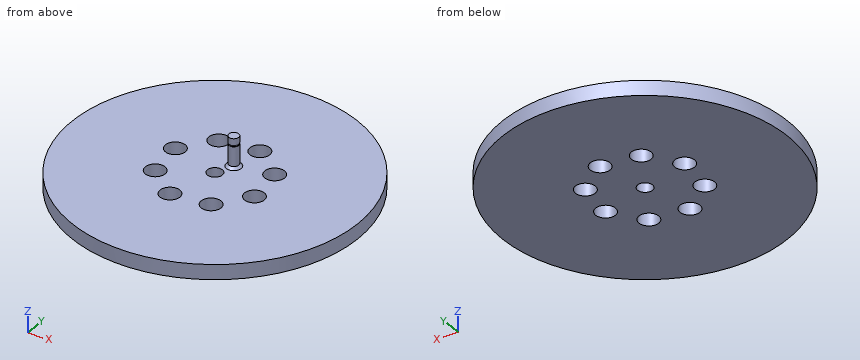
from build123d import *

# Parameters (mm, degrees)
SKETCH_1_R          = 57.5
SKETCH_1_R_2        = 3
EXTRUDE_1_DEPTH     = 6
SKETCH_3_R          = 4
CUT_EXTRUDE_2_DEPTH = 82.538334543
SKETCH_4_R          = 2
EXTRUDE_2_DEPTH     = 12
CUT_EXTRUDE_START   = -3.2
SKETCH_6_R          = 2
SKETCH_6_R_2        = 1.9
CUT_EXTRUDE_3_DEPTH = 0.5
CHAMFER_1_SIZE      = 1


with BuildPart() as part:
    # 草图1 → 凸台-拉伸1 (new body)
    with BuildSketch(Plane.XY):
        Circle(SKETCH_1_R)
        Circle(SKETCH_1_R_2, mode=Mode.SUBTRACT)
    extrude(amount=EXTRUDE_1_DEPTH)

    # 草图3 → 切除-拉伸2 (cut, through all)
    with BuildSketch(Plane(origin=(0, 0, 0), x_dir=(-1, 0, 0), z_dir=(0, 0, -1))):
        with Locations((-5.091227954, 19.341132281)):
            Circle(SKETCH_3_R)
        with Locations((10.076203981, 17.276287603)):
            Circle(SKETCH_3_R)
        with Locations((19.341132281, 5.091227954)):
            Circle(SKETCH_3_R)
        with Locations((17.276287603, -10.076203981)):
            Circle(SKETCH_3_R)
        with Locations((5.091227954, -19.341132281)):
            Circle(SKETCH_3_R)
        with Locations((-10.076203981, -17.276287603)):
            Circle(SKETCH_3_R)
        with Locations((-19.341132281, -5.091227954)):
            Circle(SKETCH_3_R)
        with Locations((-17.276287603, 10.076203981)):
            Circle(SKETCH_3_R)
    extrude(amount=-CUT_EXTRUDE_2_DEPTH, mode=Mode.SUBTRACT)

    # 草图4 → 凸台-拉伸2 (add)
    with BuildSketch(Plane.XY.offset(6)):
        with Locations((2.976659474, 6.884003078)):
            Circle(SKETCH_4_R)
    extrude(amount=EXTRUDE_2_DEPTH)

    # 草图6 → 切除-拉伸3 (cut)
    with BuildSketch(Plane.XY.offset(18).offset(CUT_EXTRUDE_START)):
        with Locations((2.976659474, 6.884003078)):
            Circle(SKETCH_6_R)
        with Locations((2.976659474, 6.884003078)):
            Circle(SKETCH_6_R_2, mode=Mode.SUBTRACT)
    extrude(amount=CUT_EXTRUDE_3_DEPTH, mode=Mode.SUBTRACT)

    # 倒角1
    chamfer_1_edges = [part.edges().sort_by_distance(p)[0] for p in [
        (0.976659474, 6.884003078, 6),
    ]]
    chamfer(chamfer_1_edges, length=CHAMFER_1_SIZE)


solid = part.part
Design review of the part built by this model. Coordinates are the model's own, in mm. Coordinates: 2 decimals unless noted, no trailing zeros. Order: outer loops, then holes, each group sorted by start corner. A loop starts at its lowest first (then second) coordinate and runs counter-clockwise, first axis right, second up. Notation, with made-up numbers: M 62,-11.5 L 95,-11.5 A30 cw 95,22.5 Z; hole C 29,35 d9. An arc over 180 degrees is marked long. Use a Markdown table: item, result.
(1) Add section D-D (z = 13.25). Give the boundary of the cut face in (x, y).
Worked answers:
| item | result |
|---|---|
| outline | C 2.98,6.88 d4 |
(2) Add section C-C (x = 26.5). Give the boundary of the cut face in (y, z), then the cut area to 3 significant figures.
Worked answers:
| item | result |
|---|---|
| outline | M -51.03,0 L 51.03,0 L 51.03,6 L -51.03,6 Z |
| area | 612 mm2 |
(3) Add section A-A (z = 2.75). Count the separate pieces of the cut face and the enclosed holes in it, then the cut area to 3 significant figures.
Worked answers:
| item | result |
|---|---|
| separate pieces | 1 |
| enclosed holes | 9 |
| area | 9,960 mm2 |
(4) Wall thickness on probe 1 along Z at (x, y) = (3, -2); probe 2 along X at (y, z) = (-22.5, 4.5); probe 3 along Y at (x, z) = (12, 5): over which ranges is each line inside the solid? List them lowest first.
Worked answers:
| item | result |
|---|---|
| probe 1 | z = 0 to 6 |
| probe 2 | x = -52.92 to -7.55, -2.64 to 52.92 |
| probe 3 | y = -56.23 to -20.78, -13.77 to 56.23 |
(5) Add section B-B (y = 25). Give the boundary of the cut face in (x, z).
Worked answers:
| item | result |
|---|---|
| outline | M -51.78,0 L 51.78,0 L 51.78,6 L -51.78,6 Z |
(6) For P1, Ø5, axis at x = -17.28, y = -10.08, coming from the -Z side; P2, Ø3, axis at x = 3, y = 7, coming from the -Z side; P3, Ø6, axis at x = -39, y = 19, coming from the +Z side; P4, Ø1.5, axis at y = 15, z = 6.5, coming from the +X side, all flat-tipped, find the tip position at first contact; note any pin that passes through.
Worked answers:
| item | result |
|---|---|
| P1 | passes through |
| P2 | stops at z = 0 |
| P3 | stops at z = 6 |
| P4 | stops at x = 55.66 |
